Study the drawing (mm; zero at the part's minimum x, y, z) and answer. A direction names the side the tool comes from. Coordinates: 2 decimals unless noted, no trailing zeros. Order: outer loops, then holes, each group sorted by start corner. A loop starts at its lowest first (then second) coordinate and runs counter-clockwise, first axis right, second up. Notation, with made-up numbers: (-25.5, -27) -> (28.5, -27) arc R11 ccw to (28.5, -21) -> close; hole circle Ø9 at (3, -39.5). An arc over 180 degrees is marked (long way). One line per question, with ' | ' between items.
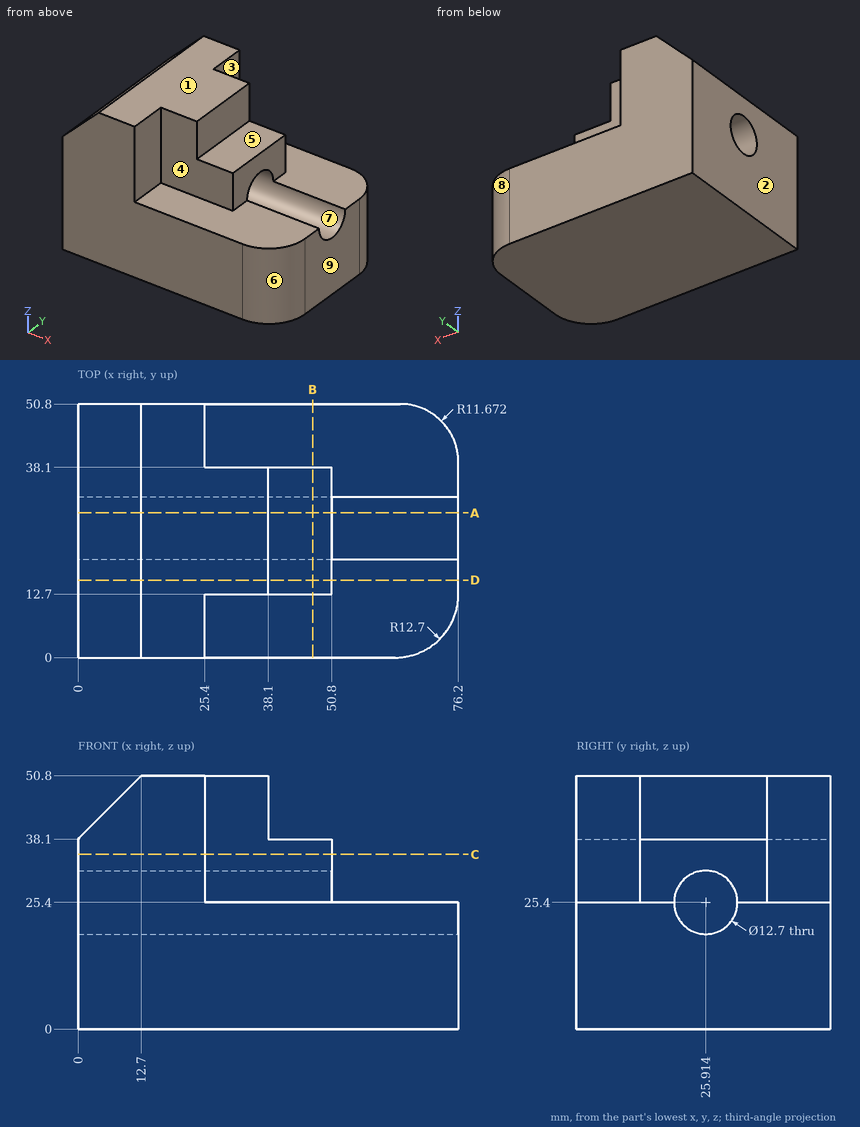
Item 1: Section D-D, the plane y = 15.5 is taken. Give the vertices of the cut face in (x, z).
Computed values:
outline: (0, 0) -> (76.2, 0) -> (76.2, 25.4) -> (50.8, 25.4) -> (50.8, 38.1) -> (38.1, 38.1) -> (38.1, 50.8) -> (12.7, 50.8) -> (0, 38.1) -> close
Item 2: Find the intervals of material crossed by L1, parallel to Y at x = 42, z = 25; L2, parallel to Z at x = 26.5, y = 26; L3, parallel to Y at x = 18, z = 23 (3 decimals), in increasing order.
Computed values:
L1: y = 0 to 19.58, 32.25 to 50.8 | L2: z = 0 to 19.05, 31.75 to 50.8 | L3: y = 0 to 20.035, 31.793 to 50.8
Item 3: Determine the mould class of the marked faces 6, 7, 8 and 9 for opening direction Y: pulls with the +Y half, pulls with the -Y half, needs draft (parallel to the pull), parting line crosses it, or undercut.
Computed values:
face 6: pulls with the -Y half | face 7: undercut | face 8: pulls with the +Y half | face 9: needs draft
Item 4: Each of these flat-tipped pins is pushed along its axis until it touches: pin 1 Ø14 at (y, z) = (3.5, 42.5) entering from +X; pin 2 Ø15.5 at (x, y) = (47, 8.5) entering from +Z; pin 3 Ø4 at (y, z) = (30, 45.5) entering from +X. Where does it stop, or does it pass through?
Computed values:
pin 1: stops at x = 25.4 | pin 2: stops at z = 38.1 | pin 3: stops at x = 38.1
Item 5: Section B-B, the plane x = 47 is taken. Give the vertices of the cut face in (y, z).
Computed values:
outline: (0, 0) -> (50.8, 0) -> (50.8, 25.4) -> (38.1, 25.4) -> (38.1, 38.1) -> (12.7, 38.1) -> (12.7, 25.4) -> (0, 25.4) -> close; hole circle Ø12.7 at (25.91, 25.4)
Item 6: Section C-C, the plane z = 35 is taken. Give the vertices of the cut face in (x, y), plus the area to 3 significant figures.
Computed values:
outline: (0, 0) -> (25.4, 0) -> (25.4, 12.7) -> (50.8, 12.7) -> (50.8, 38.1) -> (25.4, 38.1) -> (25.4, 50.8) -> (0, 50.8) -> close | area: 1,940 mm^2
Item 7: Section A-A, the plane y = 29 is taken. Give the vertices of the cut face in (x, z).
Computed values:
outline: (0, 0) -> (76.2, 0) -> (76.2, 19.85) -> (0, 19.85) -> close; (0, 30.95) -> (50.8, 30.95) -> (50.8, 38.1) -> (38.1, 38.1) -> (38.1, 50.8) -> (12.7, 50.8) -> (0, 38.1) -> close
Item 8: For the marked faces 1, 2, 3, 4 and 5, determine the directions among +Z, -Z, +X, -X, +Y, -Y from which every point of the face is accessible in a straight line to the end or side of a thin tool.
Computed values:
face 1: +Z, +X, -X, +Y, -Y | face 2: +Z, -Z, -X, +Y, -Y | face 3: +Z, +X, +Y | face 4: +Z, +X, -Y | face 5: +Z, +X, +Y, -Y
